The model under review builds one solid part; all positions refer to its coordinate system, in mm. Face numbers are marked on the shaded views. A direction names the side the tool comes from. Coordinates: 2 decimals unless noted, no trailing zeros. Write each loop counter-clockwise with the first axis right and the second up, starting at its lowest first coordinate (ties: lowest second). Pieces come first, ordered by that corner, then holes. Notation, with made-up numbers: (78, 35) - (119, 35) arc R33 ccw to (119, 63) - close; hole circle Ø3 at (39.25, -19.75). An arc over 180 degrees is marked (long way). Put each result on its own line as item: value. Start each with the question number.
Item 1: Consider section D-D on x = 10.5. Give the boundary of the cut face in (y, z), then the cut area to 3 significant figures.
Item 2: Mouldability with a two-part tool opening along X and no side actions: class the marked faces 1, 2 and 3 as pulls with the +X half, pulls with the -X half, needs draft (parallel to the pull), parting line crosses it, or undercut.
Item 3: Consider section B-B on x = 19. Give the boundary of the cut face in (y, z), then the cut area to 3 significant figures.
Item 4: To check wall thickness, follow L1, parallel to X at y = 24.25, z = 17; L2, parallel to Z at x = 1.75, y = 15; L3, parallel to Z at x = 30.5, y = 13.25. State the ranges of each line that lie inside material, in increasing order. Write a range as [from, to].
Item 5: Machinability: for the marked faces 4, 5 and 6, which of the approach directions +Z, -Z, +X, -X, +Y, -Y give a long, thin tool a straight path to every point of the face, cutting with its end or side? Answer none if there is none.
Item 6: For pin 1 (6.5 mm diameter, centred on x = 18.08, y = 14.99, fed in from +Z); pin 2 (10 mm diameter, centred on x = 8.5, z = 16, fed in from -Y); pin 3 (0.9 mm diameter, centred on x = 34, z = 9, fed in from -Y); pin 4 (0.9 mm diameter, centred on x = 35, z = 7.5, fed in from +Y), all flat-tipped, find the tip position at first contact; note any pin that passes through.
Item 7: Consider section C-C on x = 29. Give the boundary of the cut face in (y, z).
Item 8: Consider section A-A on z = 5.25. Give the boundary of the cut face in (x, y).
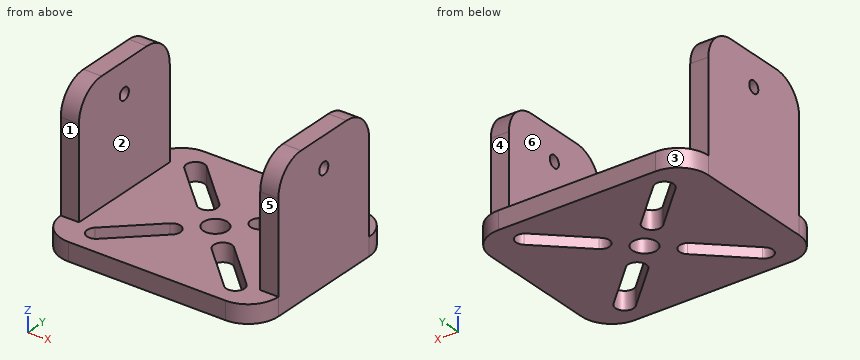
```python
from build123d import *

# Parameters (mm, degrees)
SKETCH1_W           = 36
SKETCH1_H           = 30
SKETCH1_R           = 2
BOSS_EXTRUDE2_DEPTH = 3
SKETCH2_R           = 1
BOSS_EXTRUDE3_DEPTH = 3
BOSS_EXTRUDE4_START = -3
SKETCH3_R           = 1
BOSS_EXTRUDE4_DEPTH = 3
FILLET1_R           = 5


with BuildPart() as part:
    # Sketch1 → Boss-Extrude2 (new body)
    with BuildSketch(Plane.XY):
        with Locations((18, 15)):
            Rectangle(SKETCH1_W, SKETCH1_H)
        with Locations((18.080429635, 14.989140404)):
            Circle(SKETCH1_R, mode=Mode.SUBTRACT)
        with BuildLine():
            Line((30.628958922, 24.853393036), (23.382773138, 17.961891633))
            ThreePointArc((23.382773138, 17.961891633), (21.26212006, 18.01509429), (21.315322717, 20.135747368))
            Line((21.315322717, 20.135747368), (28.561508501, 27.027248771))
            ThreePointArc((28.561508501, 27.027248771), (30.682161579, 26.974046114), (30.628958922, 24.853393036))
        make_face(mode=Mode.SUBTRACT)
        with BuildLine():
            Line((23.38198698, 12.023010255), (30.633153673, 5.136749906))
            ThreePointArc((30.633153673, 5.136749906), (30.687889624, 3.016135849), (28.567275568, 2.961399898))
            Line((28.567275568, 2.961399898), (21.316108876, 9.847660248))
            ThreePointArc((21.316108876, 9.847660248), (21.261372924, 11.968274304), (23.38198698, 12.023010255))
        make_face(mode=Mode.SUBTRACT)
        with BuildLine():
            Line((14.862197308, 9.858378688), (7.616011524, 2.966877285))
            ThreePointArc((7.616011524, 2.966877285), (5.495358446, 3.020079942), (5.548561103, 5.14073302))
            Line((5.548561103, 5.14073302), (12.794746887, 12.032234423))
            ThreePointArc((12.794746887, 12.032234423), (14.915399965, 11.979031766), (14.862197308, 9.858378688))
        make_face(mode=Mode.SUBTRACT)
        with BuildLine():
            Line((7.615225366, 26.996328337), (14.866392058, 20.110067987))
            ThreePointArc((14.866392058, 20.110067987), (14.92112801, 17.989453931), (12.800513954, 17.934717979))
            Line((12.800513954, 17.934717979), (5.549347261, 24.820978329))
            ThreePointArc((5.549347261, 24.820978329), (5.49461131, 26.941592385), (7.615225366, 26.996328337))
        make_face(mode=Mode.SUBTRACT)
    extrude(amount=BOSS_EXTRUDE2_DEPTH)

    # Sketch2 → Boss-Extrude3 (add)
    with BuildSketch(Plane(origin=(36, 0, 0), x_dir=(0, 0, -1), z_dir=(1, 0, 0))):
        with BuildLine():
            Line((-18, 5), (-3, 5))
            Line((-3, 5), (-3, 25))
            Line((-3, 25), (-18, 25))
            ThreePointArc((-18, 25), (-21.535533906, 23.535533906), (-23, 20))
            Line((-23, 20), (-23, 10))
            ThreePointArc((-23, 10), (-21.535533906, 6.464466094), (-18, 5))
        make_face()
        with Locations((-18, 15)):
            Circle(SKETCH2_R, mode=Mode.SUBTRACT)
    extrude(amount=-BOSS_EXTRUDE3_DEPTH)

    # Sketch3 → Boss-Extrude4 (add)
    with BuildSketch(Plane.ZY.offset(BOSS_EXTRUDE4_START)):
        with BuildLine():
            Line((3, 25), (18, 25))
            ThreePointArc((18, 25), (21.535533906, 23.535533906), (23, 20))
            Line((23, 20), (23, 10))
            ThreePointArc((23, 10), (21.535533906, 6.464466094), (18, 5))
            Line((18, 5), (3, 5))
            Line((3, 5), (3, 25))
        make_face()
        with Locations(Location((18, 15, 0), (0, 0, 180))):
            Circle(SKETCH3_R, mode=Mode.SUBTRACT)
    extrude(amount=BOSS_EXTRUDE4_DEPTH)

    # Fillet1
    fillet1_edges = [part.edges().sort_by_distance(p)[0] for p in [
        (36, 30, 1.5),
        (0, 30, 1.5),
        (0, 0, 1.5),
        (36, 0, 1.5),
    ]]
    fillet(fillet1_edges, radius=FILLET1_R)


solid = part.part
```
Report:
1. outline: (0, 0) - (5.71, 0) - (5.71, 3) - (0, 3) - close; (9.85, 0) - (20.12, 0) - (20.12, 3) - (9.85, 3) - close; (24.26, 0) - (30, 0) - (30, 3) - (24.26, 3) - close
1. area: 65.2 mm²
2. face 1: needs draft
2. face 2: undercut
2. face 3: pulls with the -X half
3. outline: (0, 0) - (13.21, 0) - (13.21, 3) - (0, 3) - close; (16.77, 0) - (30, 0) - (30, 3) - (16.77, 3) - close
3. area: 79.3 mm²
4. L1: [0, 3], [33, 36]
4. L2: [0, 17], [19, 23]
4. L3: [0, 3]
5. face 4: +Z, +X, -X, +Y
5. face 5: +Z, +X, -X, -Y
5. face 6: +Z, +Y, -Y
6. pin 1: z = 3
6. pin 2: through
6. pin 3: y = 5
6. pin 4: y = 25
7. outline: (0, 0) - (2.67, 0) - (2.67, 3) - (0, 3) - close; (6.69, 0) - (23.3, 0) - (23.3, 3) - (6.69, 3) - close; (27.32, 0) - (30, 0) - (30, 3) - (27.32, 3) - close
8. outline: (0, 5) - (3, 5) - (3, 25) - (0, 25) - close; (33, 5) - (36, 5) - (36, 25) - (33, 25) - close
